from build123d import *

# Parameters (mm, degrees)
F3_DEPTH = 25
F4_R     = 24.99999


# Not quite as in the source:
# - a fillet or chamfer is up to 0.001 mm smaller than in the source, because OpenCascade refuses the exact size


with BuildPart() as f1:
    # F0 (on Front) → F1 (revolve)
    with BuildSketch(Plane.XZ):
        Polygon((75, -25.5240468681), (0, -25.5240468681), (0, -40.5240468681), (90, -40.5240468681), (90, 59.4759531319), (75, 59.4759531319), align=None)
    revolve(axis=Axis((0, 0, -33.0240468681), (0, 0, -1)))

    # F2 (on Front) → F3 (join, symmetric)
    with BuildSketch(Plane.XZ):
        Polygon((83.5348658891, -40.5240468681), (93.5348658891, -40.5240468681), (93.5348658891, 116.5947673723), (34.0373912061, 176.0922420554), (26.9663233942, 169.0211742435), (83.5348658891, 112.4526317486), align=None)
    extrude(amount=F3_DEPTH, both=True)

    # F4 (radius 25 in the source; OpenCascade refuses exactly that, so slightly less here)
    f4_edges = [f1.edges().sort_by_distance(p)[0] for p in [
        (30.501857, -25, 172.556708),
        (30.501857, 25, 172.556708),
    ]]
    fillet(f4_edges, radius=F4_R)


solid = f1.part
Model file for the job. Use its own axes, mm. A direction names the side the tool comes from. Coordinates: 2 decimals unless noted, no trailing zeros. Write each loop counter-clockwise with the first axis right and the second up, starting at its lowest first coordinate (ties: lowest second). Pieces come first, ordered by that corner, then holes. Notation, with made-up numbers: (-3.75, -10.75) -> (36.25, -10.75) arc R26 ccw to (36.25, 21.25) -> close; hole circle Ø11 at (-0.75, 28). An arc over 180 degrees is marked (long way). One line per item, written item: value. Start each with the question number.
1) Flat gauge pins, fed straight in: pin 1 Ø1.5 at (x, z) = (10, 40) entering from -Y; pin 2 Ø5 at (x, z) = (41, 35.5) entering from -Y; pin 3 Ø2 at (y, z) = (-30.5, 47) entering from -X. Where does each tip first touch, or does it go through?
2) Slice it at A-A on x = -72. Write the cut outline in (y, z).
3) Slice it at D-D on y = -4. Write the cut outline in (x, z), then the cut area to 3 significant figures.
4) Slice it at C-C on x = 68.5. Write the cut outline in (y, z).
5) Probe probe 1 along Y at (x, z) = (-3, 33); probe 2 along X at (y, z) = (0, -1.5); probe 3 along Y at (x, z) = (0, 33.5). List the from-to ranges inside material, lowest first.
6) Pull direction Z, two halves, no side cores. Call faces 6 (the face through (-1, -1, -25.524)), 7 (the face through (64.2, -0.35, 145.93)), 8 (the face through (-89.928, -3.603, 10.176)): +Z half, -Z half, draft (parallel to the pull), parting line (faces both ways), or undercut.
7) Which spindle directions (+Z, -Z, +X, -X, +Y, -Y) get a long thin tool onto all of the face, cutting with end or side? Do faces 1 (the face through (35.768, -17.871, 167.191)), 2 (the face through (54.855, -0.35, 141.133)), 3 (the face through (87, 25, 74)), 4 (the face through (87, -25, 74)), 5 (the face through (35.768, 17.871, 167.191)). Say none if no direction does.
8) Slice it at B-B on z = 13. Write the cut outline in (x, y).
Answers follow:
1. pin 1: y = -89.52
1. pin 2: y = -81.35
1. pin 3: x = -85.03
2. outline: (-54, -40.52) -> (54, -40.52) -> (54, 59.48) -> (21, 59.48) -> (21, -25.52) -> (-21, -25.52) -> (-21, 59.48) -> (-54, 59.48) -> close
3. outline: (-89.91, -40.52) -> (93.53, -40.52) -> (93.53, 116.59) -> (34.27, 175.86) -> (27.19, 168.79) -> (83.53, 112.45) -> (83.53, 59.48) -> (74.89, 59.48) -> (74.89, -25.52) -> (-74.89, -25.52) -> (-74.89, 59.48) -> (-89.91, 59.48) -> close
3. area: 6,980 mm2
4. outline: (-58.38, -40.52) -> (58.38, -40.52) -> (58.38, 59.48) -> (30.54, 59.48) -> (30.54, -25.52) -> (-30.54, -25.52) -> (-30.54, 59.48) -> (-58.38, 59.48) -> close; (-25, 127.49) -> (25, 127.49) -> (25, 141.63) -> (-25, 141.63) -> close
5. probe 1: -89.95 to -74.94, 74.94 to 89.95
5. probe 2: -90 to -75, 75 to 93.53
5. probe 3: -90 to -75, 75 to 90
6. face 6: undercut
6. face 7: +Z half
6. face 8: draft
7. face 1: +Z, -X, -Y
7. face 2: -X, +Y, -Y
7. face 3: +Z, +X, +Y
7. face 4: +Z, +X, -Y
7. face 5: +Z, -X, +Y
8. outline: (86.46, -25) -> (93.53, -25) -> (93.53, 25) -> (86.46, 25) arc R90 ccw (long way) to start; hole circle Ø150 at (0, 0)
